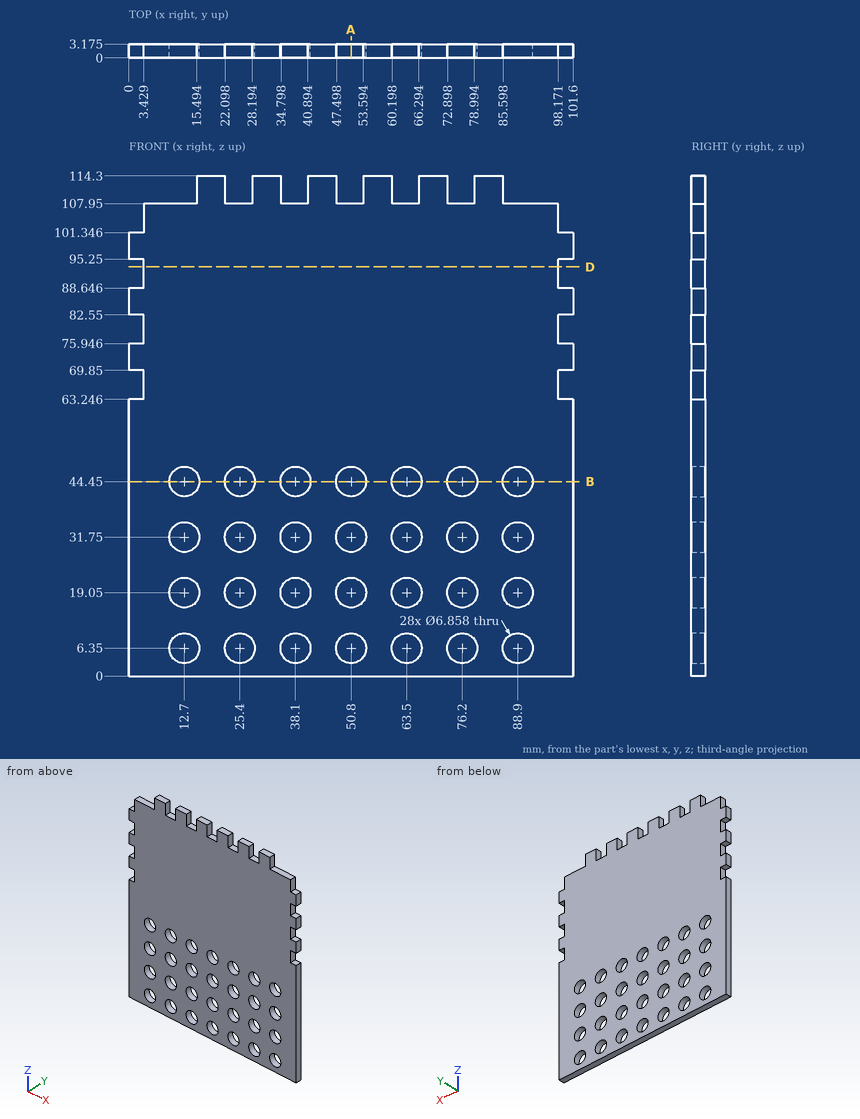
Job drawing, mm, ordinate dimensions from the low corner. One solid piece. Give positions to 0.01 mm unless a question says otherwise; leave off trailing zeros. Loops run counter-clockwise (first coordinate to the right, second up) from the corner with the lowest first, then second, coordinate; pieces in that order, holes last.
Item 1: Drill centre lines: line 1 (Z direction, x = 15, y = 1.65); line 2 (Z direction, x = 77.5, y = 2.65); line 3 (X direction, y = 1.4, z = 89). Where is each one in solid material? Low to high.
Answers follow:
line 1: z = 0 to 3.81, 8.89 to 16.51, 21.59 to 29.21, 34.29 to 41.91, 46.99 to 107.95
line 2: z = 0 to 3.18, 9.52 to 15.88, 22.22 to 28.58, 34.92 to 41.28, 47.62 to 107.95
line 3: x = 3.43 to 98.17
Item 2: Slice it at B-B, the plane z = 44.45. Give the number of separate pieces and of enclosed holes in the cut face, and give its area (3 significant figures).
Answers follow:
separate pieces: 8
enclosed holes: 0
area: 170 mm2
Item 3: Slice it at D-D, the plane z = 93.5. List the corners of the cut face in (x, y) (3 decimals), and give its area (3 significant figures).
Answers follow:
outline: (3.429, 0) - (98.171, 0) - (98.171, 3.175) - (3.429, 3.175) - close
area: 301 mm2
Item 4: Slice it at A-A, the plane x = 50.8. List the corners of the cut face in (y, z) (3 decimals).
Answers follow:
outline: (0, 0) - (3.175, 0) - (3.175, 2.921) - (0, 2.921) - close; (0, 9.779) - (3.175, 9.779) - (3.175, 15.621) - (0, 15.621) - close; (0, 22.479) - (3.175, 22.479) - (3.175, 28.321) - (0, 28.321) - close; (0, 35.179) - (3.175, 35.179) - (3.175, 41.021) - (0, 41.021) - close; (0, 47.879) - (3.175, 47.879) - (3.175, 107.95) - (0, 107.95) - close
Item 5: Flat gauge pins, fed straight in: pin 1 (1 mm diameter, centred on y = 2.5, z = 111.5, fed in from -X); pin 2 (1.6 mm diameter, centred on x = 1.5, y = 1.5, fed in from +Z). Where does each tip first touch, or does it go through?
Answers follow:
pin 1: stops at x = 15.49
pin 2: stops at z = 101.35
